```python
from build123d import *

# Parameters (mm, degrees)
BOSS_EXTRUDE1_DEPTH = 5
SKETCH2_W           = 20
SKETCH2_H           = 10
BOSS_EXTRUDE2_DEPTH = 3.75
SKETCH3_R           = 3.775
CUT_EXTRUDE1_DEPTH  = 10
SKETCH4_R           = 1.5
CUT_EXTRUDE2_DEPTH  = 5
SKETCH5_R           = 1.5
CUT_EXTRUDE3_DEPTH  = 4


with BuildPart() as part:
    # Sketch1 → Boss-Extrude1 (new body)
    with BuildSketch(Plane(origin=(0, 0, 0), x_dir=(1, 0, 0), z_dir=(0, 1, 0))):
        Polygon((-32.518521424, 35), (187.481478576, 35), (187.481478576, 15), (-32.518521424, 15), (-42.518521424, 0), (-62.518521424, 0), (-62.518521424, 20), (-42.518521424, 20), align=None)
    extrude(amount=BOSS_EXTRUDE1_DEPTH)

    # Sketch2 → Boss-Extrude2 (add)
    with BuildSketch(Plane(origin=(0, 5, 0), x_dir=(1, 0, 0), z_dir=(0, 1, 0))):
        with Locations((62.481478576, 20)):
            Rectangle(SKETCH2_W, SKETCH2_H)
    extrude(amount=BOSS_EXTRUDE2_DEPTH)

    # Sketch3 → Cut-Extrude1 (cut)
    with BuildSketch(Plane(origin=(0, 0, -25), x_dir=(-1, 0, 0), z_dir=(0, 0, -1))):
        with Locations((-62.481478576, 8.75)):
            Circle(SKETCH3_R)
    extrude(amount=-CUT_EXTRUDE1_DEPTH, mode=Mode.SUBTRACT)

    # Sketch4 → Cut-Extrude2 (cut)
    with BuildSketch(Plane(origin=(0, 5, 0), x_dir=(1, 0, 0), z_dir=(0, 1, 0))):
        with Locations(Location((182.481478576, 20, 0), (0, 0, 270))):
            Circle(SKETCH4_R)
        with Locations(Location((177.481478576, 25, 0), (0, 0, 270))):
            Circle(SKETCH4_R)
        with Locations(Location((182.481478576, 30, 0), (0, 0, 270))):
            Circle(SKETCH4_R)
        with Locations(Location((-57.518521424, 5, 0), (0, 0, 270))):
            Circle(SKETCH4_R)
        with Locations(Location((-57.518521424, 15, 0), (0, 0, 270))):
            Circle(SKETCH4_R)
        with Locations(Location((-52.518521424, 10, 0), (0, 0, 270))):
            Circle(SKETCH4_R)
    extrude(amount=-CUT_EXTRUDE2_DEPTH, mode=Mode.SUBTRACT)

    # Sketch5 → Cut-Extrude3 (cut)
    with BuildSketch(Plane(origin=(0, 8.75, 0), x_dir=(1, 0, 0), z_dir=(0, 1, 0))):
        with Locations(Location((55.481478576, 22, 0), (0, 0, 270))):
            Circle(SKETCH5_R)
        with Locations(Location((69.481478576, 18, 0), (0, 0, 270))):
            Circle(SKETCH5_R)
    extrude(amount=-CUT_EXTRUDE3_DEPTH, mode=Mode.SUBTRACT)


solid = part.part
```
The model under review builds one solid part; all positions refer to its coordinate system, in mm. A direction names the side the tool comes from. Give positions to 0.01 mm unless a question says otherwise; leave off trailing zeros. Write each loop counter-clockwise with the first axis right and the second up, starting at its lowest first coordinate (ties: lowest second). Pieces come first, ordered by that corner, then holes. Notation, with made-up numbers: M -3.5,59.25 L 3.5,59.25 A32 cw 3.5,96.25 Z; hole C 13,48.5 d5. An arc over 180 degrees is marked long. Write item = value, one per line. Start each with the question number.
Q1. Machinability: for faces 1 (the face through (-53, 2, -20)), 2 (the face through (56, 8.75, -20)), 3 (the face through (79, 2, -15)), which of the approach directions +Z, -Z, +X, -X, +Y, -Y give a long, thin tool a straight path to every point of the face, cutting with its end or side? Answer none if there is none.
Q2. For line 1 (Z direction, x = 163.5, y = 3.25); line 2 (X direction, y = 6.3, z = -22); line 3 (X direction, y = 8, z = -15.5), list the stretches that pass through material, from the lowest coordinate up.
Q3. Clearance check with flat-ended pins moving along their axes: pin 1 (3 mm diameter, centred on x = -8, z = -14.5, fed in from -Y); pin 2 (1.9 mm diameter, centred on y = 7.5, z = -19, fed in from -X); pin 3 (1.5 mm diameter, centred on y = 4, z = -14, fed in from +X); pin 4 (1.1 mm diameter, centred on x = 58.5, y = 7, fed in from -Z). State where each tip first meets the part, or that it passes through.
Q4. Mouldability with a two-part tool opening along X and no side actions: class faces 4 (the face through (-37.45, 2.46, -7.6)), 5 (the face through (64, 5, -26)), 6 (the face through (62.564, 4.976, -20.07)), 7 (the face through (-62.519, 2, -10)) as released by +X, released by -X, zero draft, split by the parting line, or undercut.
Q5. We need section A-A (y = 6.5). State the section outline as (x, z) points, plus the area to 3 significant figures.
Result set:
q1.face_1 = -Z, -X, +Y, -Y
q1.face_2 = +Z, -Z, +X, -X, +Y
q1.face_3 = +Z, +X, +Y, -Y
q2.line_1 = -35 to -15
q2.line_2 = 52.48 to 53.98, 56.98 to 59.61, 65.35 to 72.48
q2.line_3 = 52.48 to 58.78, 66.18 to 72.48
q3.pin_1 = 0
q3.pin_2 = 52.48
q3.pin_3 = -32.69
q3.pin_4 = -25
q4.face_4 = released by +X
q4.face_5 = zero draft
q4.face_6 = undercut
q4.face_7 = released by -X
q5.outline = M 52.48,-25 L 59.45,-25 L 59.45,-15 L 52.48,-15 Z; M 65.51,-25 L 72.48,-25 L 72.48,-15 L 65.51,-15 Z; hole C 55.48,-22 d3; hole C 69.48,-18 d3
q5.area = 125 mm2
